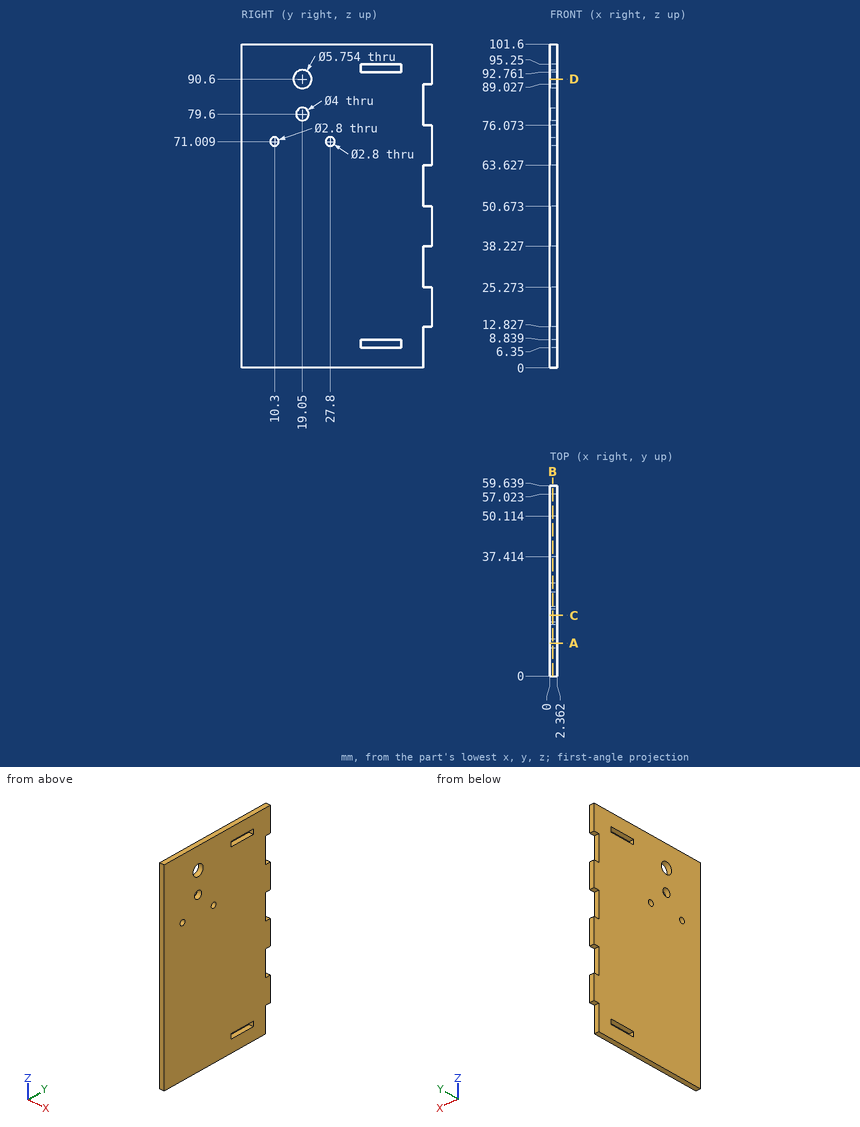
For this review, use the dimensioned drawing (mm, ordinates from the lowest corner) and the shaded views. Round coordinates to 2 decimals unless told otherwise and drop trailing zeros. Write each loop counter-clockwise with the first axis right and the second up, starting at its lowest first coordinate (ties: lowest second). Pieces come first, ordered by that corner, then holes. Notation, with made-up numbers: M 19.5,-19.75 L 28.5,-19.75 A15 cw 28.5,-10.75 Z; hole C 12.5,-24 d10. An arc over 180 degrees is marked long. Use CSV: the item, a comma, the result in double quotes. Start each with the question number.
(1) We need section D-D, the plane z = 90.6. State the section outline as (x, y) points.
(2) We need section B-B, the plane x = 0.85. State how many separate pieces and enclosed holes the cut face has, then the cut area to 3 significant figures.
(3) We need section C-C, the plane y = 19.05. State the section outline as (x, z) points.
(4) For line 1 along Z through (x, y) = (1.55, 42); line 2 along Z through (x, y) = (0.3, 20.5) (1 decimal); line 3 along Y through (x, z) = (0.7, 90.6), list the stretches that pass through material, from the lowest coordinate up.
(5) We need section A-A, the plane y = 10.3. State the section outline as (x, z) points, then the cut area to 3 significant figures.
(6) Clearance check with flat-ended pins moving along their axes: P1, Ø0.7, axis at x = 1.5, z = 59, coming from the +Y side; P2, Ø1.2, axis at x = 1.5, y = 58.5, coming from the -Z side. State where each tip first meets the part, or that it passes through.
Findings:
1,outline,"M 0,0 L 2.36,0 L 2.36,16.17 L 0,16.17 Z; M 0,21.93 L 2.36,21.93 L 2.36,59.64 L 0,59.64 Z"
2,separate pieces,"1"
2,enclosed holes,"6"
2,area,"5,810 mm^2"
3,outline,"M 0,0 L 2.36,0 L 2.36,77.6 L 0,77.6 Z; M 0,81.6 L 2.36,81.6 L 2.36,87.72 L 0,87.72 Z; M 0,93.48 L 2.36,93.48 L 2.36,101.6 L 0,101.6 Z"
4,line 1,"0 to 6.35, 8.84 to 92.76, 95.25 to 101.6"
4,line 2,"0 to 78.2, 81 to 88.1, 93.1 to 101.6"
4,line 3,"0 to 16.17, 21.93 to 59.64"
5,outline,"M 0,0 L 2.36,0 L 2.36,69.61 L 0,69.61 Z; M 0,72.41 L 2.36,72.41 L 2.36,101.6 L 0,101.6 Z"
5,area,"233 mm^2"
6,P1,"y = 57.02"
6,P2,"z = 12.83"
